Model file for the job. Use its own axes, mm. A direction names the side the tool comes from. Coordinates: 2 decimals unless noted, no trailing zeros. Order: outer loops, then holes, each group sorted by start corner. A loop starts at its lowest first (then second) coordinate and runs counter-clockwise, first axis right, second up. Notation, with made-up numbers: M 5.25,-13.75 L 15.25,-13.75 A27 cw 15.25,19.25 Z; hole C 4,-30.5 d11. An arc over 180 degrees is marked long. Return JSON: item names as keys, results as strings.
```python
from build123d import *

# Parameters (mm, degrees)
F0_W     = 35.052
F0_H     = 35.052
F1_DEPTH = 38.1
F2_R     = 1.9304
F3_DEPTH = 50.8
F4_R     = 1.27


with BuildPart() as f1:
    # F0 (on Top) → F1 (new body)
    with BuildSketch(Plane.XY):
        with Locations((-23.559753, 20.005452)):
            Rectangle(F0_W, F0_H)
    extrude(amount=F1_DEPTH)

    # F2 (on Top) → F3 (join)
    with BuildSketch(Plane.XY):
        with Locations((-23.589674, 20.671986)):
            Circle(F2_R)
    extrude(amount=F3_DEPTH)

    # F4
    f4_edges = [f1.edges().sort_by_distance(p)[0] for p in [
        (-23.559753, 37.531452, 38.1),
        (-41.085753, 37.531452, 19.05),
        (-41.085753, 2.479452, 19.05),
        (-41.085753, 20.005452, 0),
        (-41.085753, 20.005452, 38.1),
        (-23.559753, 2.479452, 38.1),
        (-6.033753, 20.005452, 38.1),
        (-6.033753, 2.479452, 19.05),
        (-23.559753, 2.479452, 0),
        (-6.033753, 37.531452, 19.05),
        (-6.033753, 20.005452, 0),
        (-23.559753, 37.531452, 0),
    ]]
    fillet(f4_edges, radius=F4_R)


solid = f1.part
```
Item 1: Saw through at A-A (x = -36). Write the cut outline in (y, z).
Check result:
{"outline": "M 2.48,1.27 A1.27 ccw 3.75,0 L 36.26,0 A1.27 ccw 37.53,1.27 L 37.53,36.83 A1.27 ccw 36.26,38.1 L 3.75,38.1 A1.27 ccw 2.48,36.83 Z"}
Item 2: Saw through at D-D (x = -24). Write the cut outline in (y, z), and give its area (3 significant figures).
Check result:
{"outline": "M 2.48,1.27 A1.27 ccw 3.75,0 L 36.26,0 A1.27 ccw 37.53,1.27 L 37.53,36.83 A1.27 ccw 36.26,38.1 L 22.56,38.1 L 22.56,50.8 L 18.79,50.8 L 18.79,38.1 L 3.75,38.1 A1.27 ccw 2.48,36.83 Z", "area": "1,380 mm2"}
Item 3: Drop flat-ended pins along their axis: pin 1 Ø2 at (x, y) = (-25.5, 10) entering from -Z; pin 2 Ø2 at (x, y) = (-12, 31.5) entering from +Z. Give the stop position or say it passes through.
Check result:
{"pin 1": "stops at z = 0", "pin 2": "stops at z = 38.1"}
Item 4: Wall check: line 1 (Z direction, x = -31, y = 24.5); line 2 (Y direction, x = -22, z = 45.5). Give the ranges that are in metal, low to high.
Check result:
{"line 1": "z = 0 to 38.1", "line 2": "y = 19.58 to 21.77"}
Item 5: Saw through at C-C (z = 40). Write the cut outline in (x, y).
Check result:
{"outline": "C -23.59,20.67 d3.86"}
Item 6: Saw through at B-B (y = 34). Write the cut outline in (x, z), and give its area (3 significant figures).
Check result:
{"outline": "M -41.09,1.27 A1.27 ccw -39.82,0 L -7.3,0 A1.27 ccw -6.03,1.27 L -6.03,36.83 A1.27 ccw -7.3,38.1 L -39.82,38.1 A1.27 ccw -41.09,36.83 Z", "area": "1,330 mm2"}
Item 7: 3-axis set-ups, long thin cutter, end or side, ignore diameter. For faces 1 (the cylindrical face through (-25.01, 21.98, 44.36)), 2 (the cylindrical face through (-6.4, 20.23, 37.72)): which of +Z, -Z, +X, -X, +Y, -Y reach the whole face in a straight line?
Check result:
{"face 1": "+Z", "face 2": "+Z, +X, +Y, -Y"}
